Input: part model. Units: mm. Frame: model coordinates. Round coordinates to 2 decimals unless told otherwise and drop trailing zeros. Loops run counter-clockwise (first coordinate to the right, second up) from the corner with the lowest first, then second, coordinate; pieces in that order, holes last. Notation, with made-up numbers: M -4.5,9 L 7.5,9 A11 ccw 7.5,26 Z; hole C -25.75,22.25 d8. An arc over 180 degrees is marked long. Put each result on its own line as item: value. Start each with the question number.
1) Section A-A on z = -10. Output: boundary loops of the cut face in (x, y), plus the area to 4 significant figures.
2) Line query: probe 1 along Z at (x, y) = (0, 1.9); probe 2 along X at (y, z) = (1.65, -10); probe 3 along X at (y, z) = (1.6, -8.5). Output: solid intervals per line, ascending.
3) Section B-B on x = 0. Output: boundary loops of the cut face in (y, z), plus the area to 3 significant figures.
4) Section C-C on y = 1.2. Output: boundary loops of the cut face in (x, z).
5) Draft query along X for faces 1 (the face through (0, 1, 15)), 2 (the face through (0.228, 1.232, 8.265)), 3 (the face through (0.228, 1.232, -11.735)), 4 (the face through (5, 1, 0)). Return one class per face: +X half, -X half, draft (parallel to the pull), parting line (faces both ways), or undercut.
Autodesk Inventor part; units mm, degrees
ref_plane "YZ Plane" through (0, 0, 0) normal (1, 0, 0) x (0, 1, 0)
ref_plane "XZ Plane" through (0, 0, 0) normal (0, 1, 0) x (-1, 0, 0)
ref_plane "XY Plane" through (0, 0, 0) normal (0, 0, 1) x (1, 0, 0)
sketch "Boceto1" plane through (0, 0, 0) normal (0, 1, 0) x (-1, 0, 0)
  circle A0 centre (0, 10) radius 1.75
  circle A1 centre (0, -10) radius 1.75
  line L0 (0, 10) -> (0, -10)
  line L1 (5, 15) -> (-5, 15)
  line L2 (-5, 15) -> (-5, -15)
  line L3 (-5, -15) -> (5, -15)
  line L4 (5, -15) -> (5, 15)
  line L5 (5, 15) -> (-5, -15) construction
  line L6 (-5, 15) -> (5, -15) construction
  point P0 (0, 0)
  point P1 (0, 0)
extrude "Extrusión1" add sketch "Boceto1" along normal blind 2.5
properties part number "standard_union"
Geometry results:
1. outline: M -5,0 L -1.75,0 L -1.75,2.5 L -5,2.5 Z; M 1.75,0 L 5,0 L 5,2.5 L 1.75,2.5 Z
1. area: 16.25 mm²
2. probe 1: z = -15 to -11.75, -8.25 to 8.25, 11.75 to 15
2. probe 2: x = -5 to -1.75, 1.75 to 5
2. probe 3: x = -5 to -0.9, 0.9 to 5
3. outline: M 0,-15 L 2.5,-15 L 2.5,-11.75 L 0,-11.75 Z; M 0,-8.25 L 2.5,-8.25 L 2.5,8.25 L 0,8.25 Z; M 0,11.75 L 2.5,11.75 L 2.5,15 L 0,15 Z
3. area: 57.5 mm²
4. outline: M -5,-15 L 5,-15 L 5,15 L -5,15 Z; hole C 0,-10 d3.5; hole C 0,10 d3.5
5. face 1: draft
5. face 2: undercut
5. face 3: undercut
5. face 4: +X half
